Part model, mm, in its own coordinate system. A direction names the side the tool comes from. Give positions to 0.01 mm unless a question says otherwise; leave off trailing zeros. Write each loop counter-clockwise with the first axis right and the second up, starting at its lowest first coordinate (ties: lowest second). Pieces come first, ordered by that corner, then holes.
Autodesk Inventor part; units mm, degrees
ref_plane "YZ Plane" through (0, 0, 0) normal (1, 0, 0) x (0, 1, 0)
ref_plane "XZ Plane" through (0, 0, 0) normal (0, 1, 0) x (-1, 0, 0)
ref_plane "XY Plane" through (0, 0, 0) normal (0, 0, 1) x (1, 0, 0)
sketch "Sketch1" plane through (0, 0, 0) normal (0, 0, 1) x (1, 0, 0)
  circle A0 centre (0, 0) radius 2.5797
  dimension "d0" = 5.1594
extrude "Extrusion1" add sketch "Sketch1" along normal blind 58.42
sketch "Sketch2" plane through (0, 0, 58.42) normal (0, 0, 1) x (1, 0, 0)
  circle A0 centre (0, 0) radius 4.1967
extrude "Extrusion2" add sketch "Sketch2" along normal blind 5.08
sketch "Sketch3" plane through (0, 0, 63.5) normal (0, 0, 1) x (1, 0, 0)
  line L0 (1.1457, 1.9844) -> (2.2914, 0)
  line L1 (2.2914, 0) -> (1.1457, -1.9844)
  line L2 (1.1457, -1.9844) -> (-1.1457, -1.9844)
  line L3 (-1.1457, -1.9844) -> (-2.2914, 0)
  line L4 (-2.2914, 0) -> (-1.1457, 1.9844)
  line L5 (-1.1457, 1.9844) -> (1.1457, 1.9844)
  point P0 (0, 0)
  point P1 (0, 0)
  point P2 (0, 1.9844)
  dimension "d5" = 3.9688
extrude "Extrusion3" cut sketch "Sketch3" against normal blind 4.445
thread "Thread1"
fillet "Fillet1" radius 0.254 1 edges at (-2.5797, 0, 0)
properties part number "10 l 20 2 1 l 2 bolt"
1) Drill centre lines: L1, parallel to Z at x = 2.75, y = -2.25; L2, parallel to Z at x = 1, y = 0 (3 decimals); L3, parallel to Y at x = -0.25, z = 28. Where is each one in solid material? Low to high.
Check result:
L1: z = 58.42 to 63.5
L2: z = 0 to 59.055
L3: y = -2.57 to 2.57
2) Mould opens along X. For faces 4 (the flat face through (-1.71, -1.01, 61.31)), 5 (the cylindrical face through (-1.901, -1.743, 28.93)), 6 (the flat face through (2, -1, 63.5)) say: +X half, -X half, draft (parallel to the pull), parting line (faces both ways), or undercut.
Check result:
face 4: undercut
face 5: parting line
face 6: draft
3) 3-axis set-ups, long thin cutter, end or side, ignore diameter. For faces 1 (the flat face through (2, 2, 58.42)), 2 (the flat face through (0, 0, 0)), 3 (the flat face through (-1.727, 0.978, 61.309)): which of +Z, -Z, +X, -X, +Y, -Y reach the whole face in a straight line?
Check result:
face 1: -Z
face 2: -Z, +X, -X, +Y, -Y
face 3: +Z
4) Saw through at B-B (z = 29.5). Write the cut outline in (x, y).
Check result:
outline: circle Ø5.16 at (0, 0)
5) Saw through at A-A (x = 0). Write the cut outline in (y, z) (3 decimals).
Check result:
outline: (-4.197, 58.42) - (-2.58, 58.42) - (-2.58, 0.254) arc R0.254 ccw to (-2.326, 0) - (2.326, 0) arc R0.254 ccw to (2.58, 0.254) - (2.58, 58.42) - (4.197, 58.42) - (4.197, 63.5) - (1.984, 63.5) - (1.984, 59.055) - (-1.984, 59.055) - (-1.984, 63.5) - (-4.197, 63.5) - close
6) Flat gauge pins, fed straight in: P1, Ø2, axis at x = 0.5, y = -2.5, coming from the -Z side; P2, Ø2, axis at x = -2, z = 23.5, coming from the +Y side; P3, Ø3, axis at y = 0.5, z = 36, coming from the +X side; P4, Ø1.5, axis at x = -1.5, z = 7.5, coming from the +Y side. Where does each tip first touch, or does it go through?
Check result:
P1: stops at z = 0
P2: stops at y = 2.38
P3: stops at x = 2.58
P4: stops at y = 2.47
